Can you work these out from the model? Positions are in its coordinate system, mm. A direction names the side the tool comes from. Coordinates: 2 decimals unless noted, no trailing zeros. Write each loop counter-clockwise with the first axis right and the second up, starting at its lowest first coordinate (ties: lowest second). Pieces come first, ordered by that corner, then holes. Notation, with made-up numbers: (57.25, -13.75) - (115.25, -13.75) arc R22 ccw to (115.25, 21.25) - close; hole circle Ø3 at (-38.75, -13). An arc over 180 degrees is marked (long way). Use one line per item in the form item = value. Start each with the question number.
(1) If we section it at B-B on y = 8: Please give me the cut outline in (x, z).
(2) On a 3-axis mill with a long thin cutter (end or side, diameter ignored), from which of +Z, -Z, +X, -X, +Y, -Y can I reach the whole of each face in a straight line? I mean faces 1 (the face through (-4.67, 6.36, -0.26)), 2 (the face through (0, 9, -3)), 3 (the face through (0, 5, 0)). Say none if no direction works.
(3) If we section it at A-A on z = 0: Please give me the cut outline in (x, y), then the cut area to 3 significant figures.
(4) If we section it at D-D on x = -5.5: Please give me the cut outline in (y, z), then the cut area to 3 significant figures.
(5) For pin 1 Ø0.8 at (x, y) = (-4.5, 4.5) entering from -Z; pin 2 Ø3 at (x, z) = (-1, 2.5) entering from +Y; pin 3 Ø1.2 at (x, z) = (-5, -1) entering from +Y; pin 4 Ø2.5 at (y, z) = (-0.5, -10) entering from -X, each with a flat end and sliding along its axis, tell me the tip position at first contact or that it passes through.
(6) If I drill on probe 1 along Y at (x, z) = (-0.75, 0); probe 2 along X at (y, z) = (6.15, 0); probe 3 along Y at (x, z) = (0.75, -9), over which ranges is the centre line in solid material (lowest first)? Write a range as from..to.
(7) Thinking about a two-plate mould opening in X: for faces 4 (the face through (0, 6, -8)), 5 (the face through (-3.86, 2.69, 1.145)), 6 (the face through (-3.5, 3.75, -1.4)), which applies, pulls with the +X half, pulls with the -X half, needs draft (parallel to the pull), parting line crosses it, or undercut?
(8) If we section it at C-C on z = 9: Please give me the cut outline in (x, y), then the cut area to 3 significant figures.
```python
from build123d import *
from build123d.topology import SkipClean

# Parameters (mm, degrees)
BASPROSKE_W                  = 10
BASPROSKE_H                  = 12
TOOTHCUT_DEPTH               = 20.697715604
TEETHCUTS_COUNT              = 10
TEETHCUTS_ANGLE              = 324
HUBNEAONESKE_R               = 7.499
HUBNEARONE_DEPTH             = 10.0000508
BORSKE_R                     = 2
BORE_DEPTH                   = 20.0000508
ESQUISSE1_W                  = 4
ESQUISSE1_H                  = 1.5
ENL_V_MAT_EXTRU_1_DEPTH      = 10
ESQUISSE8_R                  = 7.499
ENL_V_MAT_EXTRU_4_DEPTH      = 3
ENL_V_MAT_EXTRU_2_REACH      = 23.823
ENL_V_MAT_EXTRU_2_END_RADIUS = 7.499
ESQUISSE6_R                  = 1.2
ESQUISSE7_R                  = 12
ENL_V_MAT_EXTRU_3_DEPTH      = 5


with BuildPart() as part:
    # BasProSke → Base-Revolve (revolve)
    with BuildSketch(Plane(origin=(0, 0, 0), x_dir=(1, 0, 0), z_dir=(0, 1, 0)), mode=Mode.PRIVATE) as base_revolve_sk:
        with Locations((5, 6)):
            Rectangle(BASPROSKE_W, BASPROSKE_H)
    revolve(base_revolve_sk.sketch.rotate(Axis((-10, 0, 0), (1, 0, 0)), 180), axis=Axis((-10, 0, 0), (1, 0, 0)))

    # TooCutSke → ToothCut (cut, through all)
    with BuildSketch(Plane(origin=(0, 0, 0), x_dir=(0, 0, -1), z_dir=(1, 0, 0))):
        with BuildLine():
            ThreePointArc((1.173662691, 7.406586048), (0, 7.499), (-1.173662691, 7.406586048))
            ThreePointArc((-1.173662691, 7.406586048), (-1.668191438, 9.834565786), (-3.497907776, 11.50542856))
            ThreePointArc((-3.497907776, 11.50542856), (0, 12.0254), (3.497907776, 11.50542856))
            ThreePointArc((3.497907776, 11.50542856), (1.668191438, 9.834565786), (1.173662691, 7.406586048))
        make_face()
    toothcut = extrude(amount=TOOTHCUT_DEPTH, mode=Mode.SUBTRACT)

    # TeethCuts: ToothCut ×10 about axis
    teethcuts_axis = Axis((-10, 0, 0), (1, 0, 0))
    for i in range(1, TEETHCUTS_COUNT):
        add(toothcut.rotate(teethcuts_axis, i * TEETHCUTS_ANGLE / (TEETHCUTS_COUNT - 1)), mode=Mode.SUBTRACT)

    # HubNeaOneSke → HubNearOne (add)
    with SkipClean():  # the faces are left unmerged after this step: merging them gives an invalid solid
        with BuildSketch(Plane.ZY):
            Circle(HUBNEAONESKE_R)
        extrude(amount=HUBNEARONE_DEPTH)

    # BorSke → Bore (cut, symmetric)
    with SkipClean():  # the faces are left unmerged after this step: merging them gives an invalid solid
        with BuildSketch(Plane(origin=(0, 0, 0), x_dir=(0, 0, -1), z_dir=(1, 0, 0))):
            with Locations(Location((0, 0, 0), (0, 0, 180))):
                Circle(BORSKE_R)
        extrude(amount=BORE_DEPTH, both=True, mode=Mode.SUBTRACT)

    # Esquisse1 → Enlèv. mat.-Extru.1 (cut)
    with SkipClean():  # the faces are left unmerged after this step: merging them gives an invalid solid
        with BuildSketch(Plane.ZY.offset(10.0000508)):
            with Locations((0, 4.5)):
                Rectangle(ESQUISSE1_W, ESQUISSE1_H)
        extrude(amount=-ENL_V_MAT_EXTRU_1_DEPTH, mode=Mode.SUBTRACT)

    # Esquisse8 → Enlèv. mat.-Extru.4 (cut)
    with SkipClean():  # the faces are left unmerged after this step: merging them gives an invalid solid
        with BuildSketch(Plane.ZY.offset(10.0000508)):
            Circle(ESQUISSE8_R)
        extrude(amount=-ENL_V_MAT_EXTRU_4_DEPTH, mode=Mode.SUBTRACT)

    # Esquisse4 → Dégagement M21 (revolve, cut)
    with SkipClean():  # the faces are left unmerged after this step: merging them gives an invalid solid
        with BuildSketch(Plane(origin=(-3.5000508, 3.75, 0), x_dir=(0, 0, 1), z_dir=(1, 0, 0))):
            Polygon((0, 0), (0, 3.721032743), (1.2, 3), (1.2, 0), align=None)
        revolve(axis=Axis((-3.5000508, 10.1, 0), (0, -1, 0)), mode=Mode.SUBTRACT)

    # Enlèv. mat.-Extru.2: up to this cylinder (the profile starts inside it)
    with SkipClean():  # the faces are left unmerged after this step: merging them gives an invalid solid
        enl_v_mat_extru_2_end = Plane(origin=(-3.500051, 0, 0), z_dir=(-1, 0, 0)) * Cylinder(ENL_V_MAT_EXTRU_2_END_RADIUS, 63.644, mode=Mode.PRIVATE)
        # Esquisse6 → Enlèv. mat.-Extru.2 (cut, up to the surface)
        with BuildSketch(Plane(origin=(0, 3.75, 0), x_dir=(-1, 0, 0), z_dir=(0, 1, 0)), mode=Mode.PRIVATE) as enl_v_mat_extru_2_sk1:
            with Locations(Location((3.5000508, 0, 0), (0, 0, 90))):
                Circle(ESQUISSE6_R)
        enl_v_mat_extru_2_tool1 = extrude(enl_v_mat_extru_2_sk1.sketch, amount=ENL_V_MAT_EXTRU_2_REACH, mode=Mode.PRIVATE) & enl_v_mat_extru_2_end
        add(enl_v_mat_extru_2_tool1.solids().sort_by_distance((-3.500051, 3.75, 0))[0], mode=Mode.SUBTRACT)

    # Esquisse7 → Enlèv. mat.-Extru.3 (cut)
    with SkipClean():  # the faces are left unmerged after this step: merging them gives an invalid solid
        with BuildSketch(Plane(origin=(10, 0, 0), x_dir=(0, 0, -1), z_dir=(1, 0, 0))):
            Circle(ESQUISSE7_R)
        extrude(amount=-ENL_V_MAT_EXTRU_3_DEPTH, mode=Mode.SUBTRACT)


solid = part.part
```
Reported:
q1.outline = (0, -4.21) - (5, -4.21) - (5, -1.15) - (0, -1.15) - close; (0, 1.15) - (5, 1.15) - (5, 4.21) - (0, 4.21) - close
q2.face_1 = +Y
q2.face_2 = -Z, -X, +Y
q2.face_3 = -X
q3.outline = (-7, -7.5) - (5, -7.5) - (5, -2) - (-7, -2) - close; (-7, 2) - (-4.7, 2) - (-4.7, 3.75) - (-7, 3.75) - close; (-7, 5.25) - (-4.7, 5.25) - (-4.7, 7.5) - (-7, 7.5) - close; (-2.3, 2) - (5, 2) - (5, 7.5) - (-2.3, 7.5) - (-2.3, 5.25) - (0, 5.25) - (0, 3.75) - (-2.3, 3.75) - close
q3.area = 112 mm2
q4.outline = circle Ø15 at (0, 0); hole circle Ø4 at (0, 0); hole (3.75, -2) - (5.25, -2) - (5.25, 2) - (3.75, 2) - close
q4.area = 158 mm2
q5.pin_1 = -6.28
q5.pin_2 = 11.49
q5.pin_3 = 7.49
q5.pin_4 = 0
q6.probe_1 = -7.5..-2, 2..3.75, 5.25..7.5
q6.probe_2 = -7..-4.7, -2.3..5
q6.probe_3 = -7.33..-4.81, -1.53..1.53, 4.81..7.33
q7.face_4 = pulls with the -X half
q7.face_5 = undercut
q7.face_6 = needs draft
q8.outline = (0, -7.33) - (5, -7.33) - (5, -4.81) - (0, -4.81) - close; (0, -1.53) - (5, -1.53) - (5, 1.53) - (0, 1.53) - close; (0, 4.81) - (5, 4.81) - (5, 7.33) - (0, 7.33) - close
q8.area = 40.5 mm2
